For this review, take the finished solid that the model builds, in its own axes (mm). A direction names the side the tool comes from. Give positions to 0.01 mm unless a question says otherwise; leave off trailing zeros. Order: outer loops, then holes, each group sorted by start corner. A loop starts at its lowest first (then second) coordinate and runs counter-clockwise, first axis right, second up. Notation, with made-up numbers: (30.25, -27.5) - (49.25, -27.5) arc R28 ccw to (49.25, 1.5) - close; hole circle Ø9 at (85.25, 39.5). An arc over 180 degrees is marked (long way). Answer as a JSON object with one key per item and string values. Group by question number.
from build123d import *

# Parameters (mm, degrees)
CROQUIS1_R              = 20
SALIENTE_EXTRUIR1_DEPTH = 50
CROQUIS2_R              = 18
SALIENTE_EXTRUIR2_DEPTH = 35
CROQUIS3_R              = 12.5
CORTAR_EXTRUIR1_DEPTH   = 28
CORTAR_EXTRUIR2_REACH   = 91.582
CROQUIS4_R              = 8
CHAFL_N1_SIZE           = 1


with BuildPart() as part:
    # Croquis1 → Saliente-Extruir1 (new body)
    with BuildSketch(Plane.XY):
        Circle(CROQUIS1_R)
    extrude(amount=SALIENTE_EXTRUIR1_DEPTH)

    # Croquis2 → Saliente-Extruir2 (add)
    with BuildSketch(Plane.XY.offset(50)):
        Circle(CROQUIS2_R)
    extrude(amount=SALIENTE_EXTRUIR2_DEPTH)

    # Croquis3 → Cortar-Extruir1 (cut)
    with BuildSketch(Plane(origin=(0, 0, 0), x_dir=(-1, 0, 0), z_dir=(0, 0, -1))):
        Circle(CROQUIS3_R)
    extrude(amount=-CORTAR_EXTRUIR1_DEPTH, mode=Mode.SUBTRACT)

    # Croquis4 → Cortar-Extruir2 (cut, up to next)
    with BuildSketch(Plane.XY.offset(85), mode=Mode.PRIVATE) as cortar_extruir2_sk1:
        Circle(CROQUIS4_R)
    cortar_extruir2_tool1 = extrude(cortar_extruir2_sk1.sketch, amount=-CORTAR_EXTRUIR2_REACH, mode=Mode.PRIVATE) & part.part
    add(cortar_extruir2_tool1.solids().sort_by_distance((0, 0, 85))[0], mode=Mode.SUBTRACT)

    # Chaflán1
    chafl_n1_edges = [part.edges().sort_by_distance(p)[0] for p in [
        (-20, 0, 0),
        (-18, 0, 85),
    ]]
    chamfer(chafl_n1_edges, length=CHAFL_N1_SIZE)


solid = part.part
1) Consider section C-C (z = 7). Give the boundary of the cut face in (x, y).
2) Mouldability with a two-part tool opening along Y and no side actions: class faces 4 (the face through (-18, 3, 50)), 5 (the face through (-1.73, -7.81, 56.9)), 6 (the face through (-4.336, -19.524, 25.157)) as released by +Y, released by -Y, zero draft, split by the parting line, or undercut.
3) For faces 1 (the face through (12.4, -4, 0)), 2 (the face through (0.2, -8.2, 28)), 3 (the face through (-2.343, 17.847, 66.762)), list the 3-axis set-ups (+Z, -Z, +X, -X, +Y, -Y) from which the entire face can be reached by the end or side of a thin tool; tool diameter is ignored.
4) Consider section D-D (z = 33.5). Give the boundary of the cut face in (x, y).
5) For line 1 (Y direction, x = 0, z = 58); line 2 (Y direction, x = 0, z = 18); line 3 (Z direction, x = -9, y = -1), list the stretches that pass through material, from the lowest coordinate up.
6) For pin 1 (12 mm diameter, centred on y = 9, z = 30.5, fed in from +X); pin 2 (1.5 mm diameter, centred on y = 2.5, z = 37.5, fed in from +X); pin 3 (3 mm diameter, centred on x = -14.5, y = -12, fed in from +Z), all flat-tipped, find the tip position at first contact; note any pin that passes through.
7) Consider section A-A (y = 0). Give the boundary of the cut face in (x, z), plus the area to 3 significant figures.
Result set:
{
 "1": {"outline": "circle Ø40 at (0, 0); hole circle Ø25 at (0, 0)"},
 "2": {"face 4": "zero draft", "face 5": "undercut", "face 6": "split by the parting line"},
 "3": {"face 1": "-Z, +X, -X, +Y, -Y", "face 2": "-Z", "face 3": "+Z"},
 "4": {"outline": "circle Ø40 at (0, 0); hole circle Ø16 at (0, 0)"},
 "5": {"line 1": "y = -18 to -8, 8 to 18", "line 2": "y = -20 to -12.5, 12.5 to 20", "line 3": "z = 28 to 85"},
 "6": {"pin 1": "stops at x = 19.77", "pin 2": "stops at x = 19.92", "pin 3": "stops at z = 84.68"},
 "7": {"outline": "(-20, 1) - (-19, 0) - (-12.5, 0) - (-12.5, 28) - (-8, 28) - (-8, 85) - (-17, 85) - (-18, 84) - (-18, 50) - (-20, 50) - close; (8, 28) - (12.5, 28) - (12.5, 0) - (19, 0) - (20, 1) - (20, 50) - (18, 50) - (18, 84) - (17, 85) - (8, 85) - close", "area": "1,650 mm2"}
}
